Print and shaded views of the part. All mm, measured from the part's lowest x, y and z. Round coordinates to 2 decimals unless told otherwise and drop trailing zeros. Write each loop counter-clockwise with the first axis right and the second up, starting at its lowest first coordinate (ties: lowest second). Pieces come first, ordered by that corner, then holes. Notation, with made-up numbers: M -19,13 L 1,13 A9 ccw 1,28 Z; hole C -13.5,31.25 d6. An arc over 180 degrees is marked long. Write item = value, one per line. Start each with the question number.
Q1. Band-saw the part on D-D on x = 20.25. Write the cut outline in (y, z) (1 decimal).
Q2. Probe L1, parallel to X at y = 11, z = 0.75; L2, parallel to X at y = 9.5, z = 1.25 (1 decimal). List the from-to ranges inside material, lowest first.
Q3. Band-saw the part on C-C on y = 20. Write the cut outline in (x, z) (1 decimal), plus the area to 3 significant figures.
Q4. Pull direction X, two halves, no side cores. Call the marked faces 1, 2, 3 and 4: released by +X, released by -X, zero draft, split by the parting line, or undercut.
Q5. Drop flat-ended pins along their axis: P1, Ø3, axis at x = 12.5, z = 5.5, coming from the +Y side; P2, Ø4.5, axis at x = 19, y = 11, coming from the +Z side. Give the stop position or say it passes through.
Q6. Band-saw the part on A-A on x = 11. Write the cut outline in (y, z).
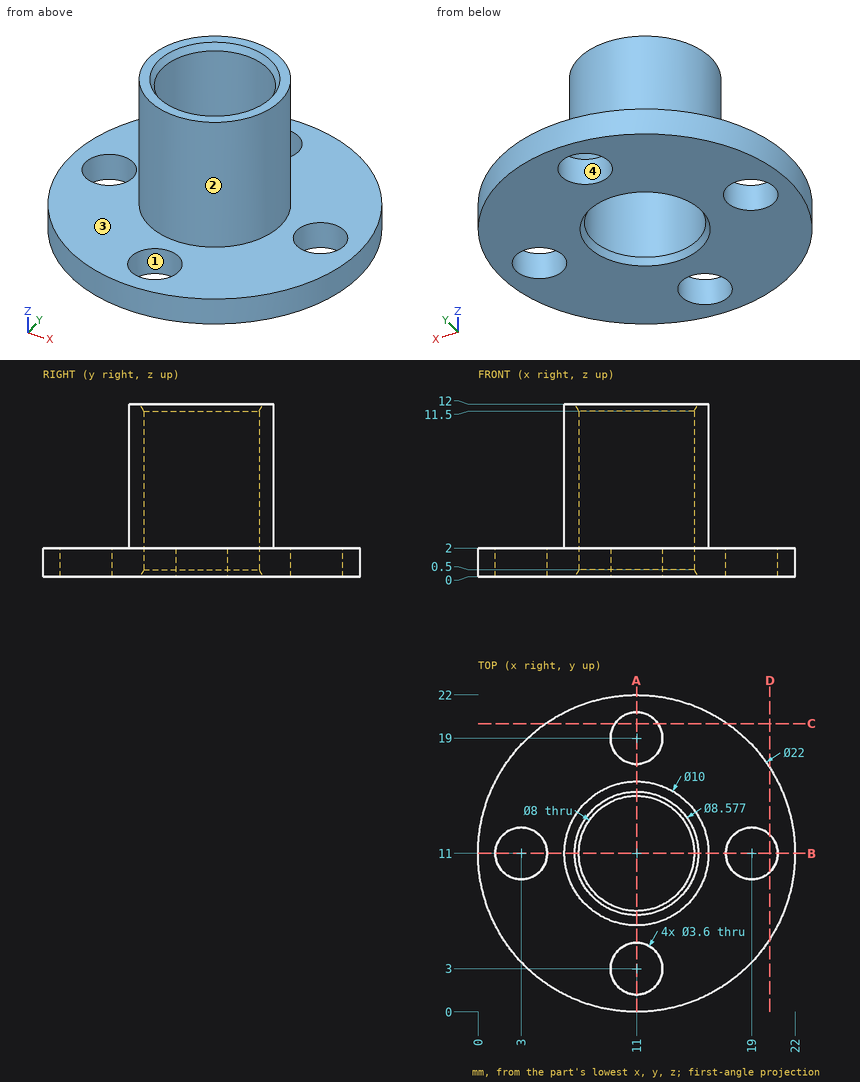
Conclusion:
q1.outline = M 5,0 L 9.7,0 L 9.7,2 L 5,2 Z; M 12.3,0 L 17,0 L 17,2 L 12.3,2 Z
q2.L1 = 0 to 1.2, 4.8 to 7, 15 to 17.2, 20.8 to 22
q2.L2 = 0.1 to 2, 4 to 7.3, 14.7 to 18, 20 to 21.9
q3.outline = M 4.7,0 L 9.5,0 L 9.5,2 L 4.7,2 Z; M 12.5,0 L 17.3,0 L 17.3,2 L 12.5,2 Z
q3.area = 19.3 mm^2
q4.face_1 = undercut
q4.face_2 = split by the parting line
q4.face_3 = zero draft
q4.face_4 = undercut
q5.P1 = 16
q5.P2 = 2
q6.outline = M 0,0 L 1.2,0 L 1.2,2 L 0,2 Z; M 4.8,0 L 6.71,0 L 7,0.5 L 7,11.5 L 6.71,12 L 6,12 L 6,2 L 4.8,2 Z; M 15,0.5 L 15.29,0 L 17.2,0 L 17.2,2 L 16,2 L 16,12 L 15.29,12 L 15,11.5 Z; M 20.8,0 L 22,0 L 22,2 L 20.8,2 Z
